```python
from build123d import *

# Parameters (mm, degrees)
F0_W      = 12
F0_H      = 22
F1_DEPTH  = 22
F3_DEPTH  = 4
F4_R      = 2.5
F5_DEPTH  = 3
F6_W      = 12
F6_H      = 3
F7_DEPTH  = 4.5
F8_W      = 12
F8_H      = 3
F9_DEPTH  = 4.5
F11_DEPTH = 3
F13_DEPTH = 3
F14_W     = 3.5
F14_H     = 1
F15_DEPTH = 2


with BuildPart() as f1:
    # F0 (on Front) → F1 (new body)
    with BuildSketch(Plane.XZ):
        Rectangle(F0_W, F0_H)
    extrude(amount=-F1_DEPTH)

    # F2 (on face) → F3 (join)
    with BuildSketch(Plane.XZ):
        with BuildLine():
            ThreePointArc((2.4451447071, -0.4791666667), (5.0334316447, 1.7343353083), (6, 5))
            ThreePointArc((6, 5), (-3.2656646917, 10.0334316447), (-2.4451447071, -0.4791666667))
            ThreePointArc((-2.4451447071, -0.4791666667), (0, 1.5), (2.4451447071, -0.4791666667))
        make_face()
        with BuildLine():
            ThreePointArc((2.4451447071, -0.4791666667), (0, 1.5), (-2.4451447071, -0.4791666667))
            ThreePointArc((-2.4451447071, -0.4791666667), (0, -1), (2.4451447071, -0.4791666667))
        make_face()
        with BuildLine():
            ThreePointArc((2.4451447071, -0.4791666667), (0, -1), (-2.4451447071, -0.4791666667))
            ThreePointArc((-2.4451447071, -0.4791666667), (-0.2618570527, -3.4862483552), (2.5, -1))
            ThreePointArc((2.5, -1), (2.4862483552, -0.7381429473), (2.4451447071, -0.4791666667))
        make_face()
    extrude(amount=F3_DEPTH)

    # F4 (on face) → F5 (join)
    with BuildSketch(Plane.XZ.offset(4)):
        with Locations((0, 5)):
            Circle(F4_R)
    extrude(amount=F5_DEPTH)

    # F6 (on face) → F7 (join)
    with BuildSketch(Plane.XY.offset(11)):
        with Locations((0, 5.5)):
            Rectangle(F6_W, F6_H)
    extrude(amount=F7_DEPTH)

    # F8 (on face) → F9 (join)
    with BuildSketch(Plane(origin=(0, 0, -11), x_dir=(1, 0, 0), z_dir=(0, 0, -1))):
        with Locations((0, -5.5)):
            Rectangle(F8_W, F8_H)
    extrude(amount=F9_DEPTH)

    # F10 (on face) → F11 (cut, through all)
    with BuildSketch(Plane.XZ.offset(-4)):
        with BuildLine():
            ThreePointArc((-0.5, 14.6456439237), (-0.6846531969, 12.4541749668), (1.25, 13.5))
            ThreePointArc((1.25, 13.5), (1.0458250332, 14.1846531969), (0.5, 14.6456439237))
            ThreePointArc((0.5, 14.6456439237), (0, 14.75), (-0.5, 14.6456439237))
        make_face()
        with BuildLine():
            ThreePointArc((-0.5, 14.6456439237), (0, 14.75), (0.5, 14.6456439237))
            Line((0.5, 14.6456439237), (0.5, 15.5))
            Line((0.5, 15.5), (-0.5, 15.5))
            Line((-0.5, 15.5), (-0.5, 14.6456439237))
        make_face()
    extrude(amount=-F11_DEPTH, mode=Mode.SUBTRACT)

    # F12 (on face) → F13 (cut, through all)
    with BuildSketch(Plane.XZ.offset(-4)):
        with BuildLine():
            ThreePointArc((0.5, -14.6456439237), (1.0458250332, -14.1846531969), (1.25, -13.5))
            ThreePointArc((1.25, -13.5), (-0.6846531969, -12.4541749668), (-0.5, -14.6456439237))
            ThreePointArc((-0.5, -14.6456439237), (0, -14.75), (0.5, -14.6456439237))
        make_face()
        with BuildLine():
            ThreePointArc((0.5, -14.6456439237), (0, -14.75), (-0.5, -14.6456439237))
            Line((-0.5, -14.6456439237), (-0.5, -15.5))
            Line((-0.5, -15.5), (0.5, -15.5))
            Line((0.5, -15.5), (0.5, -14.6456439237))
        make_face()
    extrude(amount=-F13_DEPTH, mode=Mode.SUBTRACT)

    # F14 (on face) → F15 (join)
    with BuildSketch(Plane.XY.offset(11)):
        with Locations((0, 17.5)):
            Rectangle(F14_W, F14_H)
    extrude(amount=F15_DEPTH)


solid = f1.part
```
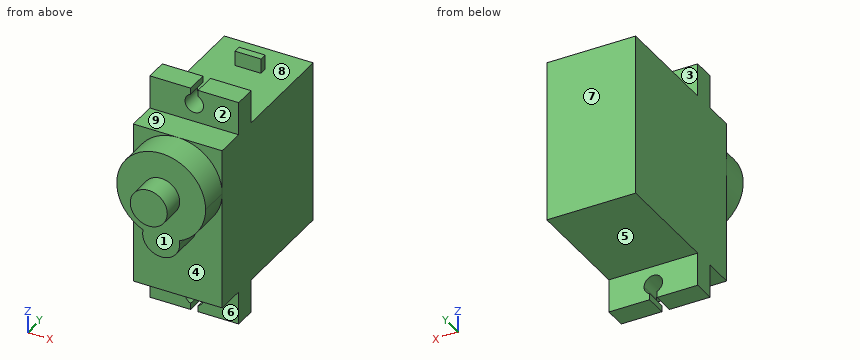
Source: CAD feature listing. Evaluate the final solid. Frame: model axes, mm. Face numbers are marked on the shaded views. A direction names the side the tool comes from. Give positions to 0.01 mm unless a question says otherwise; leave off trailing zeros. Write each loop counter-clockwise with the first axis right and the second up, starting at its lowest first coordinate (ties: lowest second). Pieces come first, ordered by that corner, then holes. Notation, with made-up numbers: (82.25, 35.5) - (109.25, 35.5) arc R14 ccw to (109.25, 49.5) - close; hole circle Ø5 at (54, -22). An arc over 180 degrees is marked (long way). One line per item, written item: value. Start each with the question number.
Q1. Material intervals for probe 1 along X at (y, z) = (5.9, 13.5); probe 2 along Y at (x, z) = (-0.5, 11.5); probe 3 along Y at (x, z) = (-4.5, 14), sorted ascending. Write a range as from..to.
Q2. Section query D-D, the plane x = -4.75. Return the cut outline in (y, z), then the cut area to 3 significant figures.
Q3. First-contact query: pin 1 Ø1 at (x, y) = (-4, 2.5) entering from +Z; pin 2 Ø2 at (x, z) = (-3, -2.5) entering from -Y; pin 3 Ø0.6 at (x, z) = (0, 11.5) entering from -Y. Flat tips, straight axial feed; report the tip coordinate or a pass-through.
Q4. Section query A-A, the plane x = 3.25. Return the cut outline in (y, z).
Q5. Section query C-C, the plane y = 3.5. Return the cut outline in (x, z), then the cut area to 3 significant figures.
Q6. Set-up query: the marked faces 1, 2, 3, 4 and 5. Return all of +Z, -Z, +X, -X, +Y, -Y with unobstructed straight access to the full face (end or side cutting, diameter ignored); none if empty.
Q7. Section query B-B, the plane z = -9. Return the cut outline in (x, y), then the cut area to 3 significant figures.
Q8. Draft query along Y for the marked faces 6, 7, 8 and 9. Return one class per face: +Y half, -Y half, draft (parallel to the pull), parting line (faces both ways), or undercut.
Answer:
1. probe 1: x = -6..-1.25, 1.25..6
1. probe 2: y = 4..7, 17..18
1. probe 3: y = 4..7
2. outline: (-4, 1.33) - (0, 1.33) - (0, -11) - (4, -11) - (4, -15.5) - (7, -15.5) - (7, -11) - (22, -11) - (22, 11) - (7, 11) - (7, 15.5) - (4, 15.5) - (4, 11) - (0, 11) - (0, 8.67) - (-4, 8.67) - close
2. area: 540 mm2
3. pin 1: stops at z = 11
3. pin 2: stops at y = -4
3. pin 3: stops at y = 4
4. outline: (-4, -0.04) - (0, -0.04) - (0, -11) - (4, -11) - (4, -15.5) - (7, -15.5) - (7, -11) - (22, -11) - (22, 11) - (7, 11) - (7, 15.5) - (4, 15.5) - (4, 11) - (0, 11) - (0, 10.04) - (-4, 10.04) - close
5. outline: (-6, -11) - (6, -11) - (6, 11) - (-6, 11) - close
5. area: 264 mm2
6. face 1: -Y
6. face 2: +Z, +X, -X, -Y
6. face 3: +Z, +X, -X
6. face 4: -Z, -Y
6. face 5: -Z, +X, -X, +Y
7. outline: (-6, 0) - (6, 0) - (6, 22) - (-6, 22) - close
7. area: 264 mm2
8. face 6: -Y half
8. face 7: +Y half
8. face 8: undercut
8. face 9: draft
